Can you work these out from the model? Positions are in its coordinate system, mm. Coordinates: 2 decimals unless noted, no trailing zeros.
Autodesk Inventor part; units mm, degrees
ref_plane "YZ Plane" through (0, 0, 0) normal (1, 0, 0) x (0, 1, 0)
ref_plane "XZ Plane" through (0, 0, 0) normal (0, 1, 0) x (-1, 0, 0)
ref_plane "XY Plane" through (0, 0, 0) normal (0, 0, 1) x (1, 0, 0)
sketch "Sketch1" plane through (0, 0, 0) normal (0, 0, 1) x (1, 0, 0)
  line L0 (0, 0) -> (20, 0)
  line L1 (20, 0) -> (20, 17.5)
  line L2 (20, 17.5) -> (0, 17.5)
  line L3 (0, 17.5) -> (0, 0)
  dimension "d0" = 20
  dimension "d1" = 17.5
extrude "Extrusion1" add sketch "Sketch1" along normal blind 1000
sketch "Sketch2" plane through (0, 17.5, 0) normal (0, 1, 0) x (1, 0, 0)
  circle A0 centre (10, -20) radius 3
  line L0 (20, 0) -> (0, 0)
  point P0 (10, 0)
  dimension "d4" = 6
  dimension "d5" = 20
extrude "Extrusion2" cut sketch "Sketch2" against normal up to surface (17.5 mm away)
sketch "Sketch3" plane through (0, 17.5, 0) normal (0, 1, 0) x (1, 0, 0)
  circle A0 centre (10, -20) radius 4.75
  circle A1 centre (10, -20) radius 3 construction
  point P0 (0, 0)
  dimension "d8" = 9.5
extrude "Extrusion3" cut sketch "Sketch3" against normal blind 8.5
pattern_linear "Rectangular Pattern1" count 18 spacing 60 along (0, 0, 1) of "Extrusion2", "Extrusion3"
properties part number "HGW20CC_Rack"
Item 1: I need wall thicknesses on line 1 along X through (y, z) = (11, 140); line 2 along X through (y, z) = (7.25, 860). Which ranges of each line are inside material? Lowest first, please.
Results are:
line 1: x = 0 to 5.25, 14.75 to 20
line 2: x = 0 to 7, 13 to 20
Item 2: Suppose I cut it at A-A, the plane x = 10. Count the separate pieces of the cut face and the enclosed holes in it, plus the area to 3 significant figures.
Results are:
separate pieces: 18
enclosed holes: 0
area: 15,200 mm2
Item 3: I'm going to push flat-ended pins straight in: P1, Ø10.5, axis at x = 8, z = 261, coming from the +Y side; P2, Ø8, axis at x = 10, z = 500, coming from the +Y side. Where does each tip first touch, or does it pass through?
Results are:
P1: stops at y = 17.5
P2: stops at y = 9
